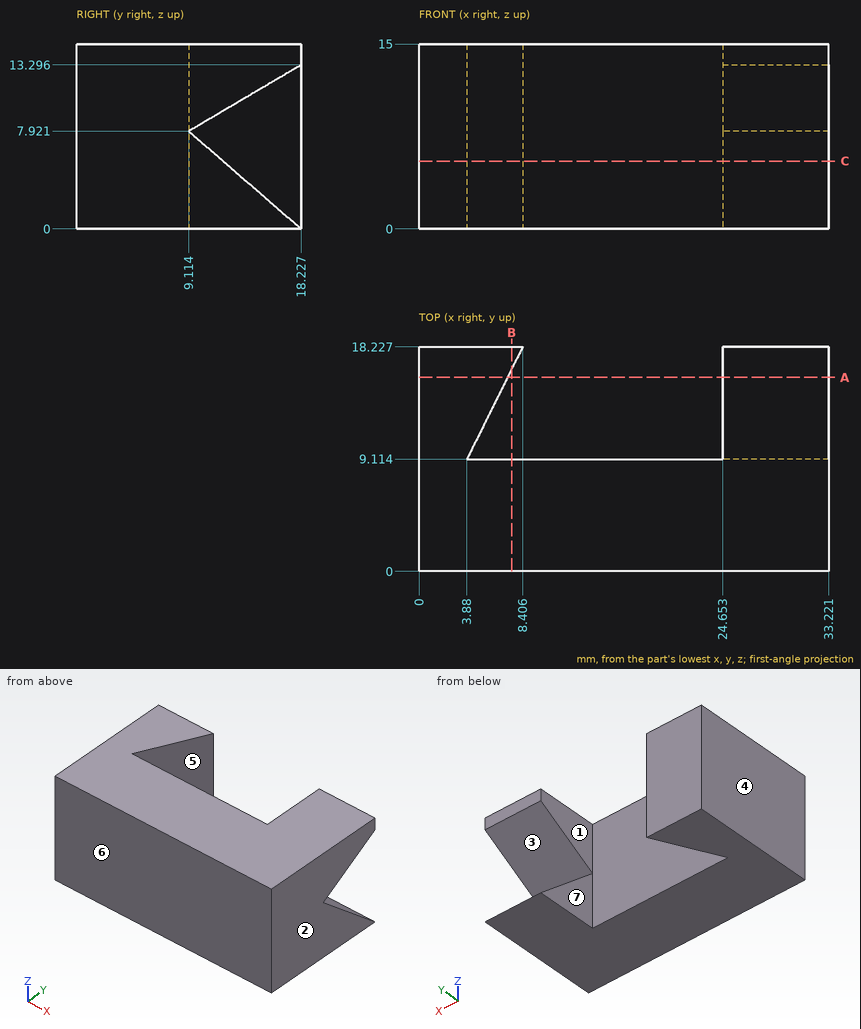
Print and shaded views of the part. All mm, measured from the part's lowest x, y and z. A direction names the side the tool comes from. Coordinates: 2 decimals unless noted, no trailing zeros. Order: outer loops, then holes, each group sorted by start corner. A loop starts at its lowest first (then second) coordinate and runs counter-clockwise, first axis right, second up. Notation, with made-up numbers: (12, 53.25) -> (16, 53.25) arc R31 cw to (16, 85.25) -> close; hole circle Ø4 at (65.25, -4.75). An arc over 180 degrees is marked (long way). Use one line per item in the form item = value. Start each with the question number.
1) Drop a flat-ended pin along its axis: pin 1 (6 mm diameter, centred on x = 27, y = 4.5, fed in from -Z). Give the stop position or say it passes through.
2) Drill centre lines: L1, parallel to Y at x = 12, z = 9.5; L2, parallel to Y at x = 4, z = 7.25 (1 decimal); L3, parallel to X at y = 10.5, z = 13.5 (1 decimal). Where is each one in solid material? Low to high. Write a range as [from, to].
3) Band-saw the part on C-C on z = 5.5. Give the cut face in (x, y).
4) Pull direction X, two halves, no side cores. Call the marked faces 1, 2, 3 and 4: +X half, -X half, draft (parallel to the pull), parting line (faces both ways), or undercut.
5) Tool access for the marked faces 5, 6 and 7: list every direction of +Z, -Z, +X, -X, +Y, -Y with a clear straight run to the whole face (end or side of a thin tool).
6) Band-saw the part on A-A on y = 15.75. Give the cut face in (x, z) (1 decimal).
7) Band-saw the part on B-B on x = 7.5. Give the cut face in (y, z), then the cut area to 3 significant figures.
Entries:
q1.pin_1 = 0
q2.L1 = [0, 9.11]
q2.L2 = [0, 9.1], [9.4, 18.2]
q2.L3 = [0, 4.6], [24.7, 33.2]
q3.outline = (0, 0) -> (33.22, 0) -> (33.22, 11.9) -> (24.65, 11.9) -> (24.65, 9.11) -> (3.88, 9.11) -> (8.41, 18.23) -> (0, 18.23) -> close
q4.face_1 = undercut
q4.face_2 = +X half
q4.face_3 = draft
q4.face_4 = -X half
q5.face_5 = +Z, -Z
q5.face_6 = +Z, -Z, +X, -X, -Y
q5.face_7 = +Z, -Z, +Y
q6.outline = (0, 0) -> (7.2, 0) -> (7.2, 15) -> (0, 15) -> close; (24.7, 0) -> (33.2, 0) -> (33.2, 2.2) -> (24.7, 2.2) -> close; (24.7, 11.8) -> (33.2, 11.8) -> (33.2, 15) -> (24.7, 15) -> close
q7.outline = (0, 0) -> (9.11, 0) -> (9.11, 15) -> (0, 15) -> close; (16.4, 0) -> (18.23, 0) -> (18.23, 15) -> (16.4, 15) -> close
q7.area = 164 mm2
